Autodesk Inventor part; units mm, degrees
ref_plane "YZ Plane" through (0, 0, 0) normal (1, 0, 0) x (0, 1, 0)
ref_plane "XZ Plane" through (0, 0, 0) normal (0, 1, 0) x (-1, 0, 0)
ref_plane "XY Plane" through (0, 0, 0) normal (0, 0, 1) x (1, 0, 0)
sketch "Sketch1" plane through (0, 0, 0) normal (0, 0, 1) x (1, 0, 0)
  line L0 (0, 0) -> (-7.5, 0)
  line L1 (-7.5, 0) -> (-7.5, 15)
  line L2 (-7.5, 15) -> (7.5, 15)
  line L3 (7.5, 15) -> (7.5, 0)
  line L4 (7.5, 0) -> (-7.5, 0)
  dimension "d55" = 7.5
  dimension "d56" = 15
  dimension "d57" = 15
extrude "Extrusion1" add sketch "Sketch1" along normal mid plane 15
sketch "Sketch11" plane through (0, 0, 7.5) normal (0, 0, 1) x (1, 0, 0)
  line L0 (7.5, 15) -> (-7.5, 15)
  line L1 (0, 15) -> (0, -25)
  line L2 (0, -25) -> (4.25, -25)
  line L3 (0, -25) -> (-4.25, -25)
  line L4 (-7.5, 0) -> (7.5, 0)
  line L5 (-4.25, -25) -> (-7.5, 0)
  line L6 (-7.5, 0) -> (7.5, 0)
  line L7 (7.5, 0) -> (4.25, -25)
  point P0 (0, 0)
  dimension "d58" = 40
  dimension "d59" = 4.25
  dimension "d60" = 4.25
extrude "Extrusion7" add sketch "Sketch11" against normal blind 15
sketch "Sketch13" plane through (0, 0, 0) normal (1, 0, 0) x (0, 1, 0)
  line L0 (15, -7.5) -> (15, 7.5)
  line L1 (15, 0) -> (-25, 0)
  line L2 (-25, 7.5) -> (-25, -7.5)
  line L3 (-25, 0) -> (-25, 4.25)
  line L4 (-25, 7.5) -> (-25, -7.5)
  line L5 (-25, 4.25) -> (-25, 0)
  line L6 (-25, 0) -> (-25, -4.25)
  line L7 (0, -7.5) -> (15, -7.5)
  line L8 (-25, -4.25) -> (0, -7.5)
  line L9 (0, -7.5) -> (0, 7.5)
  line L10 (0, 7.5) -> (-25, 4.25)
  line L11 (-25, 4.25) -> (-25, 7.5)
  line L12 (-25, 7.5) -> (0, 7.5)
  line L13 (-25, -4.25) -> (-25, -7.5)
  line L14 (-25, -7.5) -> (0, -7.5)
  line L15 (-25, -7.5) -> (0, -7.5)
  point P0 (0, 0)
  dimension "d68" = 40
  dimension "d69" = 4.25
  dimension "d70" = 4.25
extrude "Extrusion8" cut sketch "Sketch13" along normal through all both and the other way through all contours L14 L2 L8 | L10 L2 L12
sketch "Sketch15" plane through (-4.25, -25, -4.25) normal (0, -1, 0) x (1, 0, 0)
  line L0 (4.25, 4.25) -> (2.15, 4.25)
  line L1 (0, 8.5) -> (0, 0)
  line L2 (2.15, 4.25) -> (2.15, 2.15)
  line L3 (2.15, 2.15) -> (6.35, 2.15)
  line L4 (6.35, 2.15) -> (6.35, 6.35)
  line L5 (6.35, 6.35) -> (2.15, 6.35)
  line L6 (2.15, 6.35) -> (2.15, 4.25)
  point P0 (8.5, 8.5)
  point P1 (8.5, 0)
  dimension "d112" = 2.1
  dimension "d113" = 2.1
  dimension "d114" = 4.2
  dimension "d115" = 4.2
extrude "Extrusion9" cut sketch "Sketch15" against normal through all
sketch "Sketch16" plane through (0, 0, 7.5) normal (0, 0, 1) x (1, 0, 0)
  line L0 (0, 0) -> (4.9, 0)
  line L1 (-7.5, 0) -> (7.5, 0)
  line L2 (4.9, 0) -> (4.9, 16.5506)
  line L3 (0, 0) -> (-4.9, 0)
  line L4 (-4.9, 0) -> (-4.9, 16.5506)
  line L5 (-4.9, 16.5506) -> (4.9, 16.5506)
  dimension "d83" = 4.9
  dimension "d84" = 4.9
extrude "Extrusion10" cut sketch "Sketch16" against normal through all
sketch "Sketch17" plane through (7.5, 15, 7.5) normal (1, 0, 0) x (0, 0, -1)
  line L0 (15, 0) -> (0, 0)
  line L1 (0, 0) -> (7.5, 0)
  line L2 (0, 0) -> (0, -15)
  line L3 (0, -7.5) -> (0, 0)
  line L4 (0, 0) -> (15, 0)
  line L5 (15, -15) -> (15, 0)
  line L6 (15, 0) -> (15, -7.5)
  arc A0 (15, -7.5) -> (0, -7.5) centre (7.5, -7.5) ccw
  line L7 (0, -15) -> (0, 0)
  line L8 (0, -7.5) -> (0, 0)
  line L9 (15, 0) -> (0, 0)
  line L10 (0, 0) -> (15, 0)
  line L11 (15, 0) -> (15, -7.5)
  point P0 (7.5, -15)
  dimension "d133" = 15
extrude "Extrusion11" cut sketch "Sketch17" against normal through all
sketch "Sketch18" plane through (7.5, 0, 7.5) normal (1, 0, 0) x (0, 0, -1)
  line L0 (0, 0) -> (0, 15)
  line L1 (0, 15) -> (15, 15)
  line L2 (15, 15) -> (15, 0)
  line L3 (15, 0) -> (0, 0)
  line L4 (0, 15) -> (15, 0)
  line L5 (15, 15) -> (0, 0)
  circle A0 centre (7.5, 7.5) radius 4.15
  point P0 (7.5, 0)
  dimension "d90" = 15
  dimension "d91" = 8.3
extrude "Extrusion12" cut sketch "Sketch18" against normal blind 8.3 contours A0 L4 L5 | L5 L4 A0 | A0 L5 L4 | L4 L5 A0
sketch "Sketch19" plane through (-7.5, 0, -7.5) normal (-1, 0, 0) x (0, 0, 1)
  line L0 (0, 0) -> (0, 15)
  line L1 (0, 15) -> (15, 15)
  line L2 (15, 15) -> (15, 0)
  line L3 (15, 0) -> (0, 0)
  line L4 (15, 0) -> (0, 0)
  point P0 (7.5, 0)
  dimension "d94" = 15
extrude "Extrusion13" add sketch "Sketch19" along normal blind 3
sketch "Sketch20" plane through (-4.9, 0, 7.5) normal (1, 0, 0) x (0, 0, -1)
  line L0 (0, 0) -> (0, 15)
  line L1 (0, 0) -> (0, 15)
  line L2 (0, 15) -> (15, 15)
  line L3 (15, 0) -> (0, 0)
  line L4 (15, 15) -> (15, 0)
  line L5 (15, 0) -> (0, 0)
  line L6 (0, 0) -> (15, 15)
  line L7 (0, 15) -> (15, 0)
  circle A0 centre (7.5, 7.5) radius 4.15
  point P0 (7.5, 0)
  dimension "d97" = 15
  dimension "d98" = 8.3
extrude "Extrusion14" cut sketch "Sketch20" against normal blind 2.6 contours A0 L7 L6 | L6 L7 A0 | A0 L6 L7 | L7 L6 A0
sketch "Sketch21" plane through (-10.5, 0, -7.5) normal (-1, 0, 0) x (0, 0, 1)
  line L0 (0, 15) -> (0, 0)
  line L1 (15, 0) -> (15, 15)
  line L2 (0, 0) -> (15, 15)
  line L3 (0, 15) -> (0, 0)
  line L4 (15, 15) -> (0, 15)
  line L5 (0, 15) -> (15, 0)
  line L6 (7.5, 7.5) -> (7.5, 10.5)
  line L7 (7.5, 10.5) -> (10.5, 10.5)
  line L8 (10.5, 10.5) -> (10.5, 4.5)
  line L9 (10.5, 4.5) -> (4.5, 4.5)
  line L10 (4.5, 4.5) -> (4.5, 10.5)
  line L11 (4.5, 10.5) -> (10.5, 10.5)
  point P0 (7.5, 0)
  point P1 (0, 7.5)
  dimension "d101" = 3
  dimension "d102" = 3
  dimension "d103" = 6
  dimension "d104" = 6
extrude "Extrusion15" cut sketch "Sketch21" against normal blind 3 contours L11 L6 L5 | L5 L2 L10 | L2 L5 L9 | L8 L5 L2 | L2 L6 L7
sketch "Sketch23" plane through (-4.9, 0, 7.5) normal (1, 0, 0) x (0, 0, -1)
  line L0 (0, 0) -> (0, 15)
  line L1 (0, 0) -> (0, 15)
  line L2 (0, 15) -> (15, 15)
  line L3 (15, 15) -> (15, 0)
  line L4 (15, 0) -> (0, 0)
  line L5 (0, 15) -> (7.5, 15)
  arc A0 (15, 7.5) -> (0, 7.5) centre (7.5, 7.5) ccw
  line L6 (0, 7.5) -> (0, 15)
  line L7 (15, 15) -> (15, 7.5)
  point P0 (7.5, 0)
  point P1 (0, 7.5)
  dimension "d107" = 15
extrude "Extrusion16" cut sketch "Sketch23" against normal through all contours L0 L2 A0 | L2 L3 A0
fillet "Fillet2" radius 5 1 edges at (-7.5, 0, 0)
sketch "Sketch24" plane through (-10.5, 0, -7.5) normal (-1, 0, 0) x (0, 0, 1)
  line L0 (3.25, -25) -> (0, 0)
  line L1 (0, 0) -> (7.5, 0)
  line L2 (0, 0) -> (15, 0)
  line L3 (7.5, 0) -> (7.5, 4.5)
  line L4 (10.5, 4.5) -> (4.5, 4.5)
  line L5 (7.5, 4.5) -> (7.5, 7.5)
  circle A0 centre (7.5, 7.5) radius 9.5
  line L6 (1.669, 0) -> (13.331, 0)
  point P0 (13.331, 0)
  point P1 (1.669, 0)
  dimension "d116" = 3
  dimension "d117" = 19
extrude "Extrusion17" add sketch "Sketch24" along normal blind 5
sketch "Sketch25" plane through (-15.5, 0, -7.5) normal (-1, 0, 0) x (0, 0, 1)
  line L0 (0, 0) -> (1.669, 0)
  line L1 (0, 0) -> (7.5, 0)
  arc A0 (15, 1.669) -> (0, 1.669) centre (7.5, 7.5) ccw
  line L2 (7.5, 0) -> (7.5, 7.5)
  line L3 (7.5, 7.5) -> (7.5, 14.5)
  line L4 (7.5, 14.5) -> (9, 14.5)
  circle A1 centre (9, 14.5) radius 0.975
  line L5 (7.5, 7.5) -> (7.5, 0.5)
  line L6 (7.5, 0.5) -> (6, 0.5)
  line L7 (0, 0) -> (15, 0)
  circle A2 centre (6, 0.5) radius 0.975
  point P0 (13.331, 0)
  dimension "d120" = 7
  dimension "d121" = 1.5
  dimension "d122" = 1.95
  dimension "d123" = 7
  dimension "d124" = 1.5
  dimension "d125" = 90
  dimension "d126" = 1.95
extrude "Extrusion18" cut sketch "Sketch25" against normal blind 4 contours A2 L1 | L1 A2 | A1
sketch "Sketch26" plane through (-15.5, 7.5, 0) normal (-1, 0, 0) x (0, 0, 1)
  circle A0 centre (0, 0) radius 3
  point P0 (0, -7.5)
  dimension "d129" = 6
extrude "Extrusion19" cut sketch "Sketch26" against normal blind 1
equation "\"d92\" = d91"
equation "\"d105\" = d101"
properties part number "Hip joint 4 med servofeste"
Check sheet for the modelled part. Datum: model origin and axes. Units: mm. A direction names the side the tool comes from. Give positions to 0.01 mm unless a question says otherwise; leave off trailing zeros. Order: outer loops, then holes, each group sorted by start corner. A loop starts at its lowest first (then second) coordinate and runs counter-clockwise, first axis right, second up. Notation, with made-up numbers: M 51,55 L 72,55 A27 cw 72,90 Z; hole C -26.5,33 d5. An arc over 180 degrees is marked long. Answer in a Markdown table with one row per item.
1) Release check for a two-part mould opening along X. For faces 1 (the flat face through (-4.9, 4, -3)), 2 (the flat face through (-15.5, 10, -2)), 3 (the cylindrical face through (6.218, 11.615, 0.54)) record: +X half, -X half, draft (parallel to the pull), parting line (faces both ways), or undercut.
Filled sheet:
| item | result |
|---|---|
| face 1 | undercut |
| face 2 | -X half |
| face 3 | draft |
2) Thickness scan on L1, parallel to Z at x = -6.45, y = 7.5; L2, parallel to X at y = 1.5, z = 7.25; L3, parallel to Y at x = -12.85, z = 1.5 (3 decimals). Record the ranges inside material, lowest first. Write a range as [from, to].
Filled sheet:
| item | result |
|---|---|
| L1 | z = [-7.5, -4.15], [4.15, 7.5] |
| L2 | x = [-15.5, -4.9], [4.9, 7.5] |
| L3 | y = [-1.881, 13.525], [15.475, 16.881] |
3) Access from +Z, -Z, +X, -X, +Y, -Y to the whole of each face (thin tool, end or side, straight path). Record for faces 4 (the flat face through (-10.5, 0.5, -7)), 5 (the flat face through (4.9, 4, -3)), 6 (the cylindrical face through (-13.53, 0.13, -0.6)).
Filled sheet:
| item | result |
|---|---|
| face 4 | -Z, -X, -Y |
| face 5 | +Z, -Z, +Y |
| face 6 | -X |
4) Gauge pin test, flat ends, axial feed: P1, Ø2, axis at x = 6, y = 3.5, coming from the -Z side; P2, Ø10, axis at x = -2.5, y = 3.5, coming from the +Z side; P3, Ø4.5, axis at y = -14, z = 1, coming from the +X side. Record the tip position at first contact, or that the pin passes through.
Filled sheet:
| item | result |
|---|---|
| P1 | stops at z = -7.5 |
| P2 | stops at z = 7.5 |
| P3 | stops at x = 5.97 |
5) Cross-section at B-B, the plane z = 0. Count the separate pieces of the cut face and the enclosed holes in it, plus the area to 3 significant figures.
Filled sheet:
| item | result |
|---|---|
| separate pieces | 3 |
| enclosed holes | 0 |
| area | 343 mm2 |
6) Cross-section at D-D, the plane z = -3.5. Enter the section's corners in (x, y).
Filled sheet:
| item | result |
|---|---|
| outline | M -15.5,-1.33 L -10.5,-1.33 L -10.5,0 A5 cw -6.96,-4.15 L -4.25,-25 L 4.25,-25 L 7.5,0 L 7.5,5.27 L 4.9,5.27 L 4.9,0 L -4.9,0 L -4.9,5.27 L -7.5,5.27 L -7.5,9.73 L -4.9,9.73 L -4.9,14.13 L -10.5,14.13 L -10.5,16.33 L -15.5,16.33 Z; M 4.9,9.73 L 7.5,9.73 L 7.5,14.13 L 4.9,14.13 Z |
7) Cross-section at A-A, the plane y = -5. Enter the section's corners in (x, z), plus the area to 3 significant figures.
Filled sheet:
| item | result |
|---|---|
| outline | M -6.85,-6.85 L 6.85,-6.85 L 6.85,6.85 L -6.85,6.85 Z; hole M -2.1,-2.1 L 2.1,-2.1 L 2.1,2.1 L -2.1,2.1 Z |
| area | 170 mm2 |
8) Cross-section at C-C, the plane x = -13. Enter the section's corners in (y, z) (3 decimals), plus the area to 3 significant figures.
Filled sheet:
| item | result |
|---|---|
| outline | C 7.5,0 d19; hole C 0.5,-1.5 d1.95; hole C 14.5,1.5 d1.95 |
| area | 278 mm2 |
